Could you check a few things on this model? Use its own coordinates, in mm. Coordinates: 2 decimals unless noted, no trailing zeros. Loops run counter-clockwise (first coordinate to the right, second up) from the corner with the lowest first, then second, coordinate; pieces in that order, holes last.
1) Imagine slicing it at B-B on x = 23.5. Please give me the cut outline in (y, z).
2) Will these pins go through, and if not, where does the flat tip stop? P1, Ø0.8, axis at x = 25.5, z = -403, coming from the -Y side; P2, Ø1, axis at x = 22, z = -334.5, coming from the -Y side; P3, Ø4, axis at x = 23.5, z = -386, coming from the +Y side.
3) If I drill on line 1 along X through (y, z) = (52.5, -144); line 2 along Y through (x, z) = (23.75, -237); line 3 along X through (y, z) = (53, -207.5), over which ranges is the centre line in solid material (lowest first)?
4) Imagine slicing it at A-A on z = -190.5. Please give me the cut outline in (x, y).
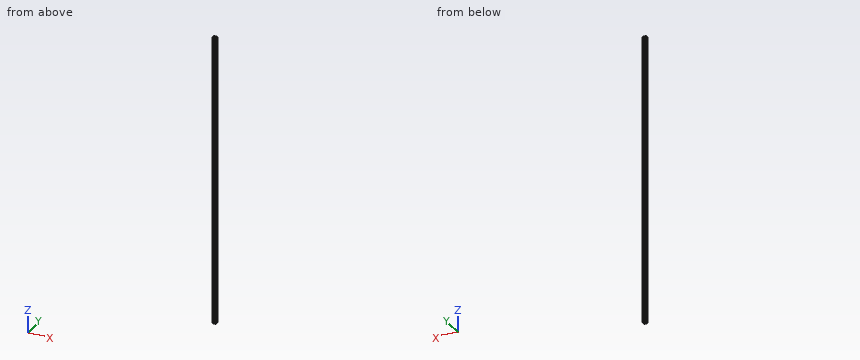
Autodesk Inventor part; units mm, degrees
ref_plane "YZ Plane" through (0, 0, 0) normal (1, 0, 0) x (0, 1, 0)
ref_plane "XZ Plane" through (0, 0, 0) normal (0, 1, 0) x (-1, 0, 0)
ref_plane "XY Plane" through (0, 0, 0) normal (0, 0, 1) x (1, 0, 0)
sketch "Boceto1" plane through (0, 0, 0) normal (0, 0, 1) x (1, 0, 0)
  line L0 (28.5, 53.7) -> (28.5, 47.2)
  line L1 (26.1, 47.2) -> (28.5, 47.2)
  line L2 (26.1, 48.45) -> (25.3942, 48.45)
  line L3 (25.3942, 48.45) -> (24.7, 47.44)
  line L4 (26.1, 52.45) -> (25.3942, 52.45)
  line L5 (26.1, 53.7) -> (28.5, 53.7)
  line L6 (24.7, 53.46) -> (25.3942, 52.45)
  line L7 (26.1, 53.7) -> (26.1, 52.45)
  line L8 (26.1, 47.2) -> (26.1, 48.45)
  line L9 (21.2, 53.46) -> (24.7, 53.46)
  line L10 (21.2, 47.44) -> (24.7, 47.44)
  line L11 (21.2, 53.46) -> (21.2, 47.44)
  point P0 (28.5, 50.45)
  dimension "d78" = 6.5
  dimension "d88" = 2.4
  dimension "d95" = 6.02
  dimension "d100" = 2.4
  dimension "d108" = 4
  dimension "d109" = 0.7058
  dimension "d110" = 0.7058
  dimension "d145" = 2
  dimension "d146" = 2
  dimension "d150" = 3.5
extrude "Extrusión1" add sketch "Boceto1" against normal blind 602
properties part number "SP40-02 JUNTA INT 207" material "Caucho, negro"
Filled in:
1. outline: (47.44, -602) - (53.46, -602) - (53.46, 0) - (47.44, 0) - close
2. P1: stops at y = 48.02
2. P2: stops at y = 47.44
2. P3: stops at y = 53.46
3. line 1: x = 21.2 to 25.36, 26.1 to 28.5
3. line 2: y = 47.44 to 53.46
3. line 3: x = 21.2 to 25.02, 26.1 to 28.5
4. outline: (21.2, 47.44) - (24.7, 47.44) - (25.39, 48.45) - (26.1, 48.45) - (26.1, 47.2) - (28.5, 47.2) - (28.5, 53.7) - (26.1, 53.7) - (26.1, 52.45) - (25.39, 52.45) - (24.7, 53.46) - (21.2, 53.46) - close
